from build123d import *

# Parameters (mm, degrees)
ESQUISSE1_R                  = 3
BOSS_EXTRU_1_DEPTH           = 93.5
ENL_V_MAT_EXTRU_1_DEPTH      = 94.596207188
ENL_V_MAT_EXTRU_1_DEPTH_BACK = 94.596207188
ESQUISSE2_R                  = 1.5
CHANFREIN1_SIZE              = 1


with BuildPart() as part:
    # Esquisse1 → Boss.-Extru.1 (new body)
    with BuildSketch(Plane.XY):
        Circle(ESQUISSE1_R)
    extrude(amount=BOSS_EXTRU_1_DEPTH)

    # Esquisse2 → Enlèv. mat.-Extru.1 (cut, two sides: drawn at the far end of the back side and taken through both)
    with BuildSketch(Plane(origin=(0, 0, 0), x_dir=(1, 0, 0), z_dir=(0, 1, 0)).offset(-ENL_V_MAT_EXTRU_1_DEPTH_BACK)):
        with Locations(Location((0, -3, 0), (0, 0, 270))):
            Circle(ESQUISSE2_R)
    extrude(amount=ENL_V_MAT_EXTRU_1_DEPTH + ENL_V_MAT_EXTRU_1_DEPTH_BACK, mode=Mode.SUBTRACT)

    # Chanfrein1
    chanfrein1_edges = [part.edges().sort_by_distance(p)[0] for p in [
        (-3, 0, 93.5),
    ]]
    chamfer(chanfrein1_edges, length=CHANFREIN1_SIZE)


solid = part.part
Design review of the part built by this model. Coordinates are the model's own, in mm. Give positions to 0.01 mm unless a question says otherwise; leave off trailing zeros. Write each loop counter-clockwise with the first axis right and the second up, starting at its lowest first coordinate (ties: lowest second). Pieces come first, ordered by that corner, then holes. Notation, with made-up numbers: M -27,-33.75 L 9,-33.75 A22 cw 9,-2.75 Z; hole C 39,-20 d7. An arc over 180 degrees is marked long. Answer as a JSON object with one key per item and string values. Group by question number.
1) We need section B-B (z = 3). Give the boundary of the cut face in (x, y).
2) Mouldability with a two-part tool opening along Z and no side actions: class faces 1 (the face through (1.265, -0.042, 3.806)), 2 (the face through (0, 0, 0)), 3 (the face through (0, 0, 93.5)) as released by +Z, released by -Z, zero draft, split by the parting line, or undercut.
3) Clearance check with a flat-ended pin moving along its axis: pin 1 Ø1.5 at (y, z) = (2, 49) entering from -X. State where the tip first meets the part, or that it passes through.
4) For line 1 along X through (y, z) = (0.25, 3); line 2 along X through (y, z) = (-1.5, 3); line 3 along Y through (x, z) = (-0.25, 55.5), list the stretches that pass through material, from the lowest coordinate up.
5) We need section A-A (x = 0). Give the boundary of the cut face in (y, z).
Answer key:
{
 "1": {"outline": "M -1.5,-2.6 L -1.5,2.6 A3 ccw Z; M 1.5,-2.6 A3 ccw 1.5,2.6 Z"},
 "2": {"face 1": "undercut", "face 2": "released by -Z", "face 3": "released by +Z"},
 "3": {"pin 1": "stops at x = -2.73"},
 "4": {"line 1": "x = -2.99 to -1.5, 1.5 to 2.99", "line 2": "x = -2.6 to -1.5, 1.5 to 2.6", "line 3": "y = -2.99 to 2.99"},
 "5": {"outline": "M -3,0 L 3,0 L 3,1.5 L -3,1.5 Z; M -3,4.5 L 3,4.5 L 3,92.5 L 2,93.5 L -2,93.5 L -3,92.5 Z"}
}
